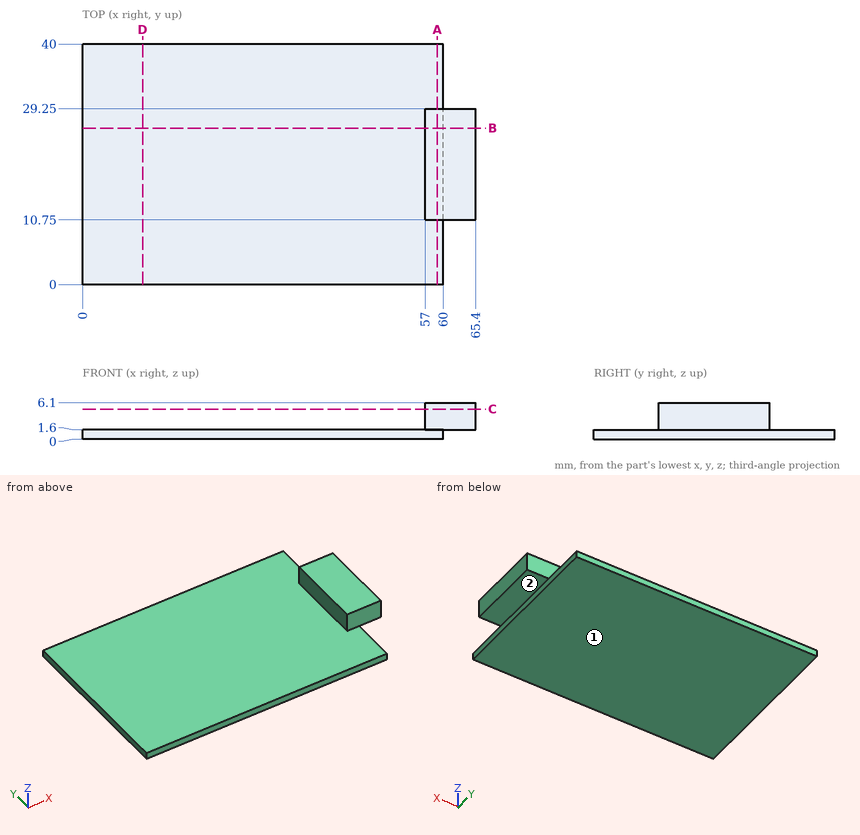
For this review, use the dimensioned drawing (mm, ordinates from the lowest corner) and the shaded views. A direction names the side the tool comes from. Coordinates: 2 decimals unless noted, no trailing zeros. Write each loop counter-clockwise with the first axis right and the second up, starting at its lowest first coordinate (ties: lowest second). Pieces come first, ordered by that corner, then holes. Notation, with made-up numbers: (7.25, -3) - (11.25, -3) arc R31 cw to (11.25, 30) - close; hole circle Ø10 at (27, -19). An arc over 180 degrees is marked (long way). Answer in a Markdown table with one row per item. Add a question column.
Q1. For the marked faces 1 and 2, list the 3-axis set-ups (+Z, -Z, +X, -X, +Y, -Y) from which the entire face can be reached by the end or side of a thin tool; tool diameter is ignored.
Q2. To check wall thickness, follow line 1 along Y through (x, z) = (58.5, 3.5); line 2 along X through (y, z) = (21.5, 5); line 3 along Z through (x, y) = (46, 35). State the ranges of each line that lie inside material, in increasing order. Write a range as from..to.
Q3. Consider section B-B on y = 26. Give the boundary of the cut face in (x, z), then the cut area to 3 significant figures.
Q4. Clearance check with flat-ended pins moving along their axes: pin 1 (1.8 mm diameter, centred on y = 20, z = 0.5, fed in from +X); pin 2 (2 mm diameter, centred on y = 24, z = 4.5, fed in from -X); pin 3 (6 mm diameter, centred on x = 15.5, y = 4.5, fed in from +Z). State where each tip first meets the part, or that it passes through.
Q5. Consider section A-A on x = 59. Give the boundary of the cut face in (y, z), then the cut area to 3 significant figures.
Q6. Consider section D-D on x = 10. Give the boundary of the cut face in (y, z).
Q7. Consider section C-C on z = 5. Give the boundary of the cut face in (x, y), then the cut area to 3 significant figures.
Answers below:
| question | item | result |
|---|---|---|
| 1 | face 1 | -Z, +X, -X, +Y, -Y |
| 1 | face 2 | -Z, +X, +Y, -Y |
| 2 | line 1 | 10.75..29.25 |
| 2 | line 2 | 57..65.4 |
| 2 | line 3 | 0..1.6 |
| 3 | outline | (0, 0) - (60, 0) - (60, 1.6) - (65.4, 1.6) - (65.4, 6.1) - (57, 6.1) - (57, 1.6) - (0, 1.6) - close |
| 3 | area | 134 mm² |
| 4 | pin 1 | x = 60 |
| 4 | pin 2 | x = 57 |
| 4 | pin 3 | z = 1.6 |
| 5 | outline | (0, 0) - (40, 0) - (40, 1.6) - (29.25, 1.6) - (29.25, 6.1) - (10.75, 6.1) - (10.75, 1.6) - (0, 1.6) - close |
| 5 | area | 147 mm² |
| 6 | outline | (0, 0) - (40, 0) - (40, 1.6) - (0, 1.6) - close |
| 7 | outline | (57, 10.75) - (65.4, 10.75) - (65.4, 29.25) - (57, 29.25) - close |
| 7 | area | 155 mm² |
